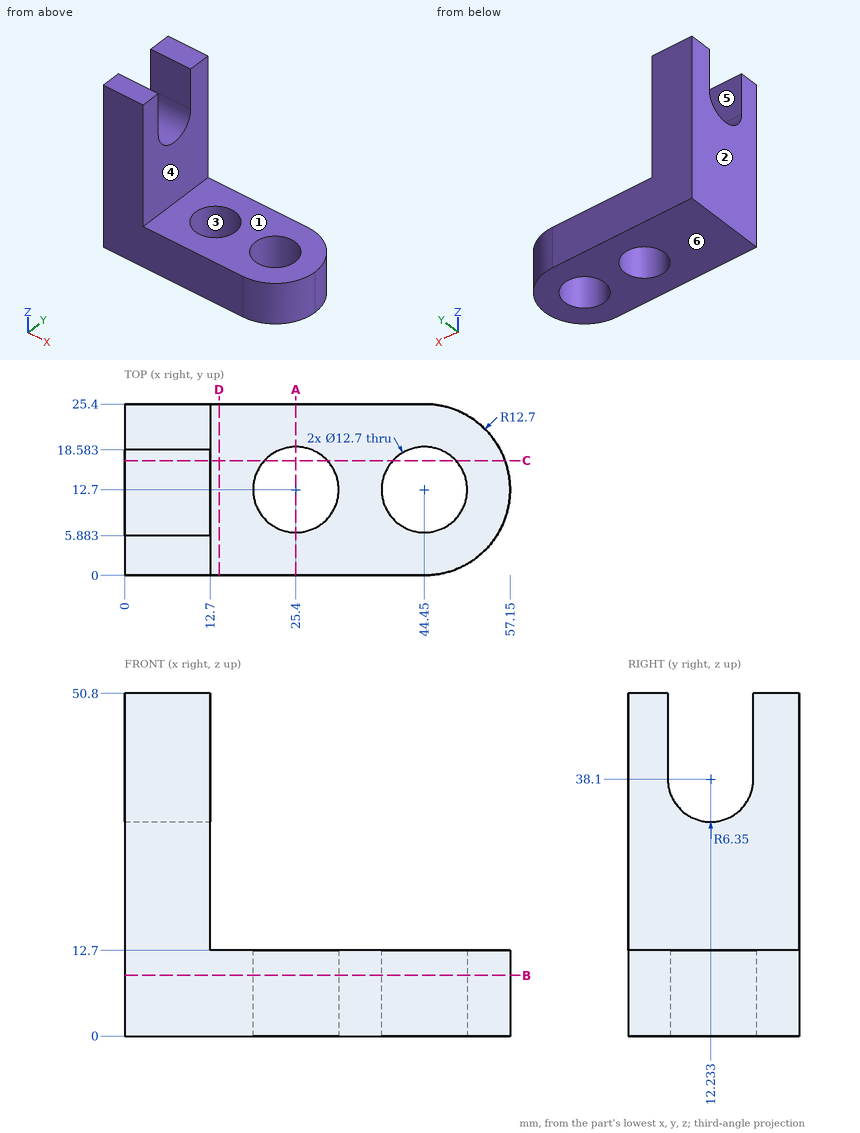
Verification items for this drawing (mm, ordinates from the low corner). A direction names the side the tool comes from. Round coordinates to 2 decimals unless told otherwise and drop trailing zeros. Loops run counter-clockwise (first coordinate to the right, second up) from the corner with the lowest first, then second, coordinate; pieces in that order, holes last. Notation, with made-up numbers: (-30.5, 17) - (23.5, 17) arc R16 cw to (23.5, 35) - close; hole circle Ø5 at (71, -29). An arc over 180 degrees is marked (long way). Write item = value, one per line.
Q1. Sectioned sample at D-D on x = 14. Record the boundary of the cut face in (y, z), plus the area to 3 significant figures.
Here are the results:
outline = (0, 0) - (25.4, 0) - (25.4, 12.7) - (0, 12.7) - close
area = 323 mm^2
Q2. Mould release check, pull along X, two halves, no side actions. Record for the marked faces 1, 2 and 3: +X half, -X half, draft (parallel to the pull), parting line (faces both ways), or undercut.
Here are the results:
face_1 = draft
face_2 = -X half
face_3 = undercut
Q3. Tool access check on the marked faces 4, 5 and 6. Record the directions out of +Z, -Z, +X, -X, +Y, -Y that give a thin tool (end or side, any length) a straight path to the whole face; none if there is none.
Here are the results:
face_4 = +Z, +X, +Y, -Y
face_5 = +Z, +X, -X
face_6 = -Z, +X, -X, +Y, -Y
Q4. Sectioned sample at A-A on x = 25.4. Record the boundary of the cut face in (y, z), plus the area to 3 significant figures.
Here are the results:
outline = (0, 0) - (6.35, 0) - (6.35, 12.7) - (0, 12.7) - close; (19.05, 0) - (25.4, 0) - (25.4, 12.7) - (19.05, 12.7) - close
area = 161 mm^2
Q5. Material ranges on L1, parallel to Y at x = 25, z = 3; L2, parallel to X at y = 13.75, z = 29.5, recorded low to high.
Here are the results:
L1 = 0 to 6.36, 19.04 to 25.4
L2 = 0 to 12.7
Q6. Depth check by flat-ended pin: pin 1 (11.5 mm diameter, centred on x = 25.4, y = 12.7, fed in from +Z); pin 2 (5 mm diameter, centred on x = 37.5, y = 6.5, fed in from +Z); pin 3 (8 mm diameter, centred on y = 6, z = 39.5, fed in from +X). Enter the tip coordinate at first touch or a pass-through.
Here are the results:
pin_1 = through
pin_2 = 12.7
pin_3 = 12.7
Q7. Sectioned sample at B-B on z = 9. Record the boundary of the cut face in (x, y).
Here are the results:
outline = (0, 0) - (44.45, 0) arc R12.7 ccw to (57.15, 12.7) arc R12.7 ccw to (44.45, 25.4) - (0, 25.4) - close; hole circle Ø12.7 at (25.4, 12.7); hole circle Ø12.7 at (44.45, 12.7)
Q8. Sectioned sample at C-C on y = 17. Record the boundary of the cut face in (x, z) (1 decimal), plus the area to 3 significant figures.
Here are the results:
outline = (0, 0) - (20.7, 0) - (20.7, 12.7) - (12.7, 12.7) - (12.7, 33.9) - (0, 33.9) - close; (30.1, 0) - (39.8, 0) - (39.8, 12.7) - (30.1, 12.7) - close; (49.1, 0) - (56.4, 0) - (56.4, 12.7) - (49.1, 12.7) - close
area = 748 mm^2
